The listing builds one solid part. Answer for the finished solid, in the listing's coordinates (mm). Face numbers are marked on the shaded views. A direction names the side the tool comes from. Give positions to 0.01 mm unless a question says otherwise; leave off trailing zeros. Loops run counter-clockwise (first coordinate to the right, second up) from the corner with the lowest first, then second, coordinate; pieces in that order, holes last. Notation, with made-up numbers: (11, -21) - (25, -21) arc R25 ccw to (25, 2) - close; hole circle Ø7 at (59, 29.5). An arc over 180 degrees is marked (long way). One line per item, written item: value. Start each with the question number.
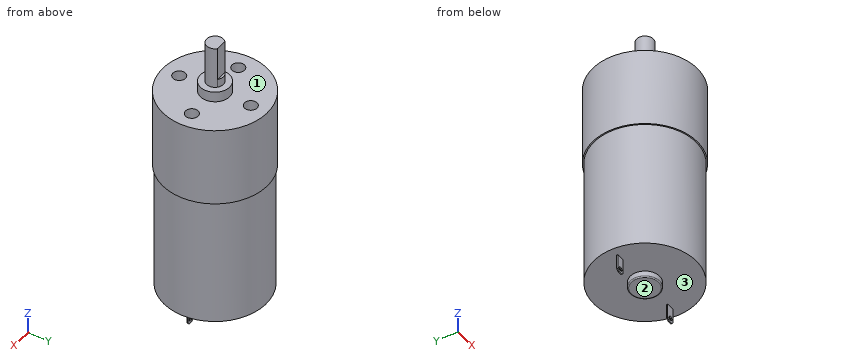
from build123d import *
from build123d.topology import SkipClean

# Parameters (mm, degrees)
SKETCH1_R                    = 12.5
BOSS_EXTRUDE1_DEPTH          = 19
SKETCH2_R                    = 12.2
BOSS_EXTRUDE2_DEPTH          = 30.8
SKETCH3_R                    = 1.5
CUT_EXTRUDE1_DEPTH           = 10
CIRPATTERN1_COUNT            = 4
SKETCH4_R                    = 3.5
BOSS_EXTRUDE3_DEPTH          = 2.5
BOSS_EXTRUDE4_DEPTH          = 10
SKETCH7_R                    = 2
BOSS_EXTRUDE5_DEPTH          = 2
SKETCH8_W                    = 2
SKETCH8_H                    = 0.25
BOSS_EXTRUDE6_DEPTH          = 4
CHAMFER1_SIZE                = 0.5
CUT_EXTRUDE2_REACH           = 58.658
SKETCH10_R                   = 0.5
CIRPATTERN2_COUNT            = 2
CHAMFER1_OF_CIRPATTERN2_SIZE = 0.5
BOSS_EXTRUDE7_START          = 1.5
SKETCH11_R                   = 3.5
BOSS_EXTRUDE7_DEPTH          = 1.5
FILLET1_R                    = 0.25


with BuildPart() as part:
    # Sketch1 → Boss-Extrude1 (new body)
    with BuildSketch(Plane.XY):
        Circle(SKETCH1_R)
    extrude(amount=-BOSS_EXTRUDE1_DEPTH)

    # Sketch2 → Boss-Extrude2 (add)
    with BuildSketch(Plane(origin=(0, 0, -19), x_dir=(-1, 0, 0), z_dir=(0, 0, -1))):
        with Locations(Location((0, 0, 0), (0, 0, 180))):
            Circle(SKETCH2_R)
    extrude(amount=BOSS_EXTRUDE2_DEPTH)

    # Sketch3 → Cut-Extrude1 (cut)
    with BuildSketch(Plane.XY):
        with Locations((-8.5, 0)):
            Circle(SKETCH3_R)
    cut_extrude1 = extrude(amount=-CUT_EXTRUDE1_DEPTH, mode=Mode.SUBTRACT)

    # CirPattern1: Cut-Extrude1 ×4 about axis
    cirpattern1_axis = Axis((0, 0, 0), (0, 0, 1))
    for i in range(1, CIRPATTERN1_COUNT):
        add(cut_extrude1.rotate(cirpattern1_axis, i * 360 / CIRPATTERN1_COUNT), mode=Mode.SUBTRACT)

    # Sketch4 → Boss-Extrude3 (add)
    with BuildSketch(Plane.XY):
        Circle(SKETCH4_R)
    extrude(amount=BOSS_EXTRUDE3_DEPTH)

    # Sketch6 → Boss-Extrude4 (add)
    with BuildSketch(Plane.XY.offset(2.5)):
        with BuildLine():
            Line((-1.322875656, 1.5), (1.322875656, 1.5))
            ThreePointArc((1.322875656, 1.5), (0, -2), (-1.322875656, 1.5))
        make_face()
    extrude(amount=BOSS_EXTRUDE4_DEPTH)

    # Sketch7 → Boss-Extrude5 (add)
    with SkipClean():  # the faces are left unmerged after this step: merging them gives an invalid solid
        with BuildSketch(Plane.XY.offset(2.5)):
            with Locations(Location((0, 0, 0), (0, 0, 131.409622109))):
                Circle(SKETCH7_R)
        extrude(amount=BOSS_EXTRUDE5_DEPTH)

    # Sketch8 → Boss-Extrude6 (add)
    with SkipClean():  # the faces are left unmerged after this step: merging them gives an invalid solid
        with BuildSketch(Plane(origin=(0, 0, -49.8), x_dir=(-1, 0, 0), z_dir=(0, 0, -1))):
            with Locations((-9.15, 0)):
                Rectangle(SKETCH8_W, SKETCH8_H)
        boss_extrude6 = extrude(amount=BOSS_EXTRUDE6_DEPTH)

    # Chamfer1
    chamfer1_edges = [part.edges().sort_by_distance(p)[0] for p in [
        (10.15, 0, -53.8),
        (8.15, 0, -53.8),
    ]]
    chamfer(chamfer1_edges, length=CHAMFER1_SIZE)

    # Sketch10 → Cut-Extrude2 (cut, up to next)
    with BuildSketch(Plane(origin=(0, 0.125, 0), x_dir=(1, 0, 0), z_dir=(0, 1, 0)), mode=Mode.PRIVATE) as cut_extrude2_sk1:
        with Locations(Location((9.15, 52.8, 0), (0, 0, 270))):
            Circle(SKETCH10_R)
    cut_extrude2_tool1 = extrude(cut_extrude2_sk1.sketch, amount=-CUT_EXTRUDE2_REACH, mode=Mode.PRIVATE) & part.part
    cut_extrude2 = cut_extrude2_tool1.solids().sort_by_distance((9.15, 0.125, -52.8))[0]
    add(cut_extrude2, mode=Mode.SUBTRACT)

    # CirPattern2: Boss-Extrude6, Cut-Extrude2 ×2 about axis
    with SkipClean():  # the faces are left unmerged after this step: merging them gives an invalid solid
        cirpattern2_axis = Axis((0, 0, 0), (0, 0, 1))
        add([boss_extrude6.rotate(cirpattern2_axis, i * 360 / CIRPATTERN2_COUNT) for i in range(1, CIRPATTERN2_COUNT)])
        add([cut_extrude2.rotate(cirpattern2_axis, i * 360 / CIRPATTERN2_COUNT) for i in range(1, CIRPATTERN2_COUNT)], mode=Mode.SUBTRACT)

    # Chamfer1 of CirPattern2
    chamfer1_of_cirpattern2_edges = [part.edges().sort_by_distance(p)[0] for p in [
        (-10.15, 0, -53.8),
        (-8.15, 0, -53.8),
    ]]
    chamfer(chamfer1_of_cirpattern2_edges, length=CHAMFER1_OF_CIRPATTERN2_SIZE)

    # Sketch11 → Boss-Extrude7 (add)
    with SkipClean():  # the faces are left unmerged after this step: merging them gives an invalid solid
        with BuildSketch(Plane(origin=(0, 0, -49.8), x_dir=(-1, 0, 0), z_dir=(0, 0, -1)).offset(BOSS_EXTRUDE7_START)):
            with Locations(Location((0, 0, 0), (0, 0, 180))):
                Circle(SKETCH11_R)
        extrude(amount=-BOSS_EXTRUDE7_DEPTH)

    # Fillet1
    fillet1_edges = [part.edges().sort_by_distance(p)[0] for p in [
        (-3.5, 0, -51.3),
    ]]
    fillet(fillet1_edges, radius=FILLET1_R)


solid = part.part
1. A cutting plane is placed at B-B (y = 8.75). Determine the outline of the cut face in (x, z).
2. For the marked faces 1, 2 and 3, determine the directions among +Z, -Z, +X, -X, +Y, -Y from which every point of the face is accessible in a straight line to the end or side of a thin tool.
3. A cutting plane is placed at A-A (z = -2.5). Determine the outline of the cut face in (x, y), plus the area to 3 significant figures.
4. Find the intervals of material crossed by L1, parallel to X at y = 0.05, z = -52.8; L2, parallel to Y at x = -7, z = -20.5; L3, parallel to Z at x = -9.15, y = 0, in increasing order. Write a range as [from, to].
5. Flat-ended cylindrical pins translate along their axes: pin 1 (3.5 mm diameter, centred on x = 0, y = 8.5, fed in from +Z); pin 2 (6 mm diameter, centred on x = 9.5, z = -17, fed in from -Y); pin 3 (1 mm diameter, centred on x = 9.5, z = -52.5, fed in from +Y) (3 decimals). Find the tip coordinate at first contact, or state that the pin passes through.
6. A cutting plane is placed at D-D (y = -9). Determine the outline of the cut face in (x, z), plus the area to 3 significant figures.
7. A cutting plane is placed at C-C (x = 4.75). Determine the outline of the cut face in (y, z), plus the area to 3 significant figures.
Results below:
1. outline: (-8.93, -19) - (-8.5, -19) - (-8.5, -49.8) - (8.5, -49.8) - (8.5, -19) - (8.93, -19) - (8.93, 0) - (1.48, 0) - (1.48, -10) - (-1.48, -10) - (-1.48, 0) - (-8.93, 0) - close
2. face 1: +Z
2. face 2: -Z, +Y, -Y
2. face 3: -Z
3. outline: circle Ø25 at (0, 0); hole circle Ø3 at (-8.5, 0); hole circle Ø3 at (0, -8.5); hole circle Ø3 at (0, 8.5); hole circle Ø3 at (8.5, 0)
3. area: 463 mm^2
4. L1: x = [-10.15, -9.65], [-8.65, -8.15], [8.15, 8.65], [9.65, 10.15]
4. L2: y = [-9.99, 9.99]
4. L3: z = [-53.8, -53.3], [-52.3, -10]
5. pin 1: stops at z = 0
5. pin 2: stops at y = -10.68
5. pin 3: stops at y = 0.125
6. outline: (-8.67, -19) - (-8.24, -19) - (-8.24, -49.8) - (8.24, -49.8) - (8.24, -19) - (8.67, -19) - (8.67, 0) - (1.41, 0) - (1.41, -10) - (-1.41, -10) - (-1.41, 0) - (-8.67, 0) - close
6. area: 809 mm^2
7. outline: (-11.56, -19) - (-11.24, -19) - (-11.24, -49.8) - (11.24, -49.8) - (11.24, -19) - (11.56, -19) - (11.56, 0) - (-11.56, 0) - close
7. area: 1,130 mm^2
